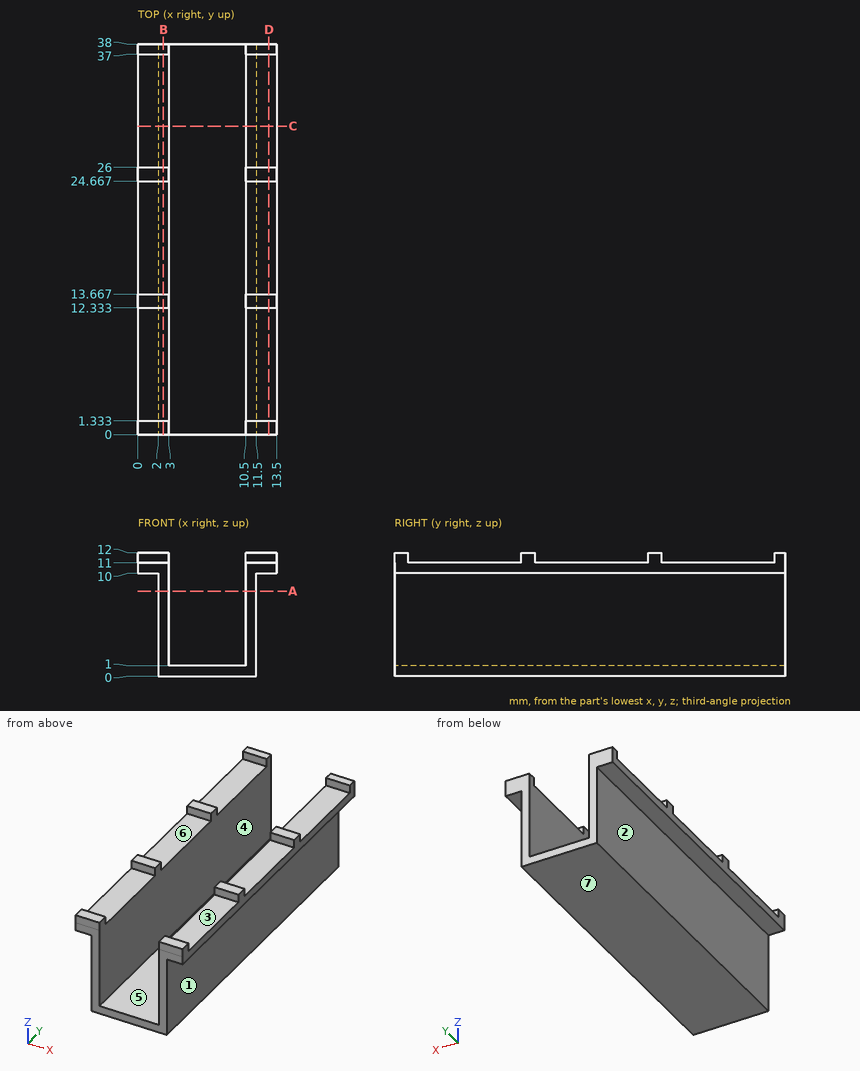
Verification items for this drawing (mm, ordinates from the low corner). A direction names the side the tool comes from. Round coordinates to 2 decimals unless told otherwise and drop trailing zeros. Loops run counter-clockwise (first coordinate to the right, second up) from the corner with the lowest first, then second, coordinate; pieces in that order, holes last. Notation, with made-up numbers: (57.25, 83) - (77.25, 83) arc R29 cw to (77.25, 105) - close; hole circle Ø10 at (-2.75, 66.5). An arc over 180 degrees is marked (long way). Write item = value, one per line.
Q1. Material ranges on L1, parallel to X at y = 14, z = 5.25; L2, parallel to Z at x = 2.5, y = 24; L3, parallel to Z at x = 5.25, y = 28, recorded low to high.
Here are the results:
L1 = 2 to 3, 10.5 to 11.5
L2 = 0 to 11
L3 = 0 to 1
Q2. Sectioned sample at D-D on x = 12.75. Record the boundary of the cut face in (y, z).
Here are the results:
outline = (0, 10) - (38, 10) - (38, 12) - (37, 12) - (37, 11) - (26, 11) - (26, 12) - (24.67, 12) - (24.67, 11) - (13.67, 11) - (13.67, 12) - (12.33, 12) - (12.33, 11) - (1.33, 11) - (1.33, 12) - (0, 12) - close
Q3. Sectioned sample at B-B on x = 2.5. Record the boundary of the cut face in (y, z).
Here are the results:
outline = (0, 0) - (38, 0) - (38, 12) - (37, 12) - (37, 11) - (26, 11) - (26, 12) - (24.67, 12) - (24.67, 11) - (13.67, 11) - (13.67, 12) - (12.33, 12) - (12.33, 11) - (1.33, 11) - (1.33, 12) - (0, 12) - close
Q4. Depth check by flat-ended pin: pin 1 (0.6 mm diameter, centred on x = 1.5, y = 13, fed in from -Z); pin 2 (4 mm diameter, centred on y = 18, z = 7, fed in from +X); pin 3 (3.5 mm diameter, centred on x = 11.5, y = 5, fed in from +Z). Enter the tip coordinate at first touch or a pass-through.
Here are the results:
pin_1 = 10
pin_2 = 11.5
pin_3 = 11
Q5. Sectioned sample at C-C on y = 30. Record the boundary of the cut face in (x, z), plus the area to 3 significant figures.
Here are the results:
outline = (0, 10) - (2, 10) - (2, 0) - (11.5, 0) - (11.5, 10) - (13.5, 10) - (13.5, 11) - (10.5, 11) - (10.5, 1) - (3, 1) - (3, 11) - (0, 11) - close
area = 33.5 mm^2
Q6. Tool access check on the marked faces 5, 6 and 7. Record the directions out of +Z, -Z, +X, -X, +Y, -Y that give a thin tool (end or side, any length) a straight path to the whole face; none if there is none.
Here are the results:
face_5 = +Z, +Y, -Y
face_6 = +Z, +X, -X
face_7 = -Z, +X, -X, +Y, -Y
Q7. Sectioned sample at A-A on z = 8.25. Record the boundary of the cut face in (x, y).
Here are the results:
outline = (2, 0) - (3, 0) - (3, 38) - (2, 38) - close; (10.5, 0) - (11.5, 0) - (11.5, 38) - (10.5, 38) - close
Q8. Mould release check, pull along X, two halves, no side actions. Record for the marked faces 1, 2, 3 and 4: +X half, -X half, draft (parallel to the pull), parting line (faces both ways), or undercut.
Here are the results:
face_1 = +X half
face_2 = -X half
face_3 = draft
face_4 = undercut
